from build123d import *

# Parameters (mm, degrees)
F0_R = 25.4
F2_R = 31.75
F4_T = -2.54


# Not quite as in the source:
# - a fillet or chamfer that OpenCascade refuses, or shapes differently, is made with other operations: its cross-section is extruded or revolved along the edge and cut away or added


with BuildPart() as f3:
    # F0 (on Top) → F3 section 0
    with BuildSketch(Plane.XY):
        Circle(F0_R)
    # F2 (on offset) → F3 section 1
    with BuildSketch(Plane.XY.offset(59.436)):
        Circle(F2_R)
    loft()

    # F4
    f4_openings = [f3.faces().sort_by_distance(p)[0] for p in [
        (0, 0, 59.436),
    ]]
    offset(amount=F4_T, openings=f4_openings, kind=Kind.INTERSECTION)

    # F5: fillet of radius 5.08 on 1 edges, made by hand

    # F5_s1 → F5_t2 (revolve, cut)
    with BuildSketch(Plane.XZ):
        with BuildLine():
            ThreePointArc((31.2538092028, 54.7916541382), (30.8469014644, 57.3895821842), (29.195545003, 59.436))
            Line((29.195545003, 59.436), (31.75, 59.436))
            Line((31.75, 59.436), (31.2538092028, 54.7916541382))
        make_face()
    revolve(axis=Axis((0, 0, 59.436), (0, 0, 1)), mode=Mode.SUBTRACT)


solid = f3.part
CAD build for the part. Positions are in the model's coordinates, mm. Round coordinates to 2 decimals unless told otherwise and drop trailing zeros. Order: outer loops, then holes, each group sorted by start corner. A loop starts at its lowest first (then second) coordinate and runs counter-clockwise, first axis right, second up. Notation, with made-up numbers: (41.25, 72) -> (91.25, 72) arc R20 cw to (91.25, 96) -> close; hole circle Ø11 at (27, 64.25). An arc over 180 degrees is marked (long way). Write item = value, one per line. Start each with the question number.
(1) Pull direction X, two halves, no side cores. Call faces 1 (the conical face through (13.09, -25.167, 27.779)), 2 (the flat face through (0, 0, 0)), 3 (the flat face through (0, 0, 2.54)): released by +X, released by -X, zero draft, split by the parting line, or undercut.
(2) Cut at B-B, the plane z = 19.5. List the corners of the cut face in (x, y), then the cut area to 3 significant figures.
(3) Cut at C-C, the plane z = 35. List the corners of the cut face in (x, y).
(4) Pin check, flat tips, straight feed: P1, Ø1.5, axis at x = 9, y = -8.5, coming from the +Z side; P2, Ø1, axis at x = 5, z = 52.5, coming from the +Y side; P3, Ø8, axis at y = -15.5, z = 14, coming from the -X side. Stop position of each tip, or through.
(5) Probe line 1 (Z direction, x = -3, y = -10); line 2 (X direction, y = 15.5, z = 44); line 3 (X direction, y = 9.5, z = 32). List the from-to ranges inside material, lowest first. Write a range as [from, to].
(6) Cut at A-A, the plane x = 0. List the corners of the cut face in (y, z).
Model answer:
q1.face_1 = split by the parting line
q1.face_2 = zero draft
q1.face_3 = undercut
q2.outline = circle Ø54.97 at (0, 0); hole circle Ø49.86 at (0, 0)
q2.area = 421 mm2
q3.outline = circle Ø58.28 at (0, 0); hole circle Ø53.17 at (0, 0)
q4.P1 = 2.54
q4.P2 = 30.7
q4.P3 = -24.37
q5.line_1 = [0, 2.54]
q5.line_2 = [-25.8, -22.77], [22.77, 25.8]
q5.line_3 = [-27.21, -24.49], [24.49, 27.21]
q6.outline = (-31.25, 54.79) -> (-25.4, 0) -> (25.4, 0) -> (31.25, 54.79) arc R5.08 ccw to (29.2, 59.44) -> (23.12, 2.54) -> (-23.12, 2.54) -> (-29.2, 59.44) arc R5.08 ccw to start
